Verification items for this drawing (mm, ordinates from the low corner). A direction names the side the tool comes from. Coordinates: 2 decimals unless noted, no trailing zeros. Order: outer loops, then holes, each group sorted by start corner. A loop starts at its lowest first (then second) coordinate and runs counter-clockwise, first axis right, second up. Notation, with made-up numbers: M -24.5,65.5 L -6.5,65.5 A23 cw -6.5,83.5 Z; hole C -22,26 d2. An arc over 180 degrees is marked long. Return JSON: item names as keys, results as strings. Group by question number.
1. Mould release check, pull along Z, two halves, no side actions. Record for the marked faces 3 and 4: +Z half, -Z half, draft (parallel to the pull), parting line (faces both ways), or undercut.
2. Section check B-B, the plane z = 13.9. Record the cut outline in (x, y).
3. Section check A-A, the plane x = 13.9. Record the cut outline in (y, z).
4. Material ranges on line 1 along Y through (x, z) = (10, 25.25); line 2 along X through (y, z) = (34, 14); line 3 along Y through (x, z) = (8.75, 20.75), recorded low to high.
5. Set-up check for the marked faces 1 and 2: record each of +Z, -Z, +X, -X, +Y, -Y from which the full face is reachable in a straight line by a thin tool's end or side.
6. Gauge pin test, flat ends, axial feed: pin 1 (4 mm diameter, centred on x = 8.24, z = 19.56, fed in from +Y); pin 2 (2.5 mm diameter, centred on x = 19.56, z = 8.24, fed in from -Y); pin 3 (4 mm diameter, centred on y = 6.5, z = 21.5, fed in from +X). Record the tip position at first contact, or that the pin passes through.
7. Section check C-C, the plane y = 14. Record the cut outline in (x, z), plus the area to 3 significant figures.
8. Section check D-D, the plane x = 24.75. Record the cut outline in (y, z).
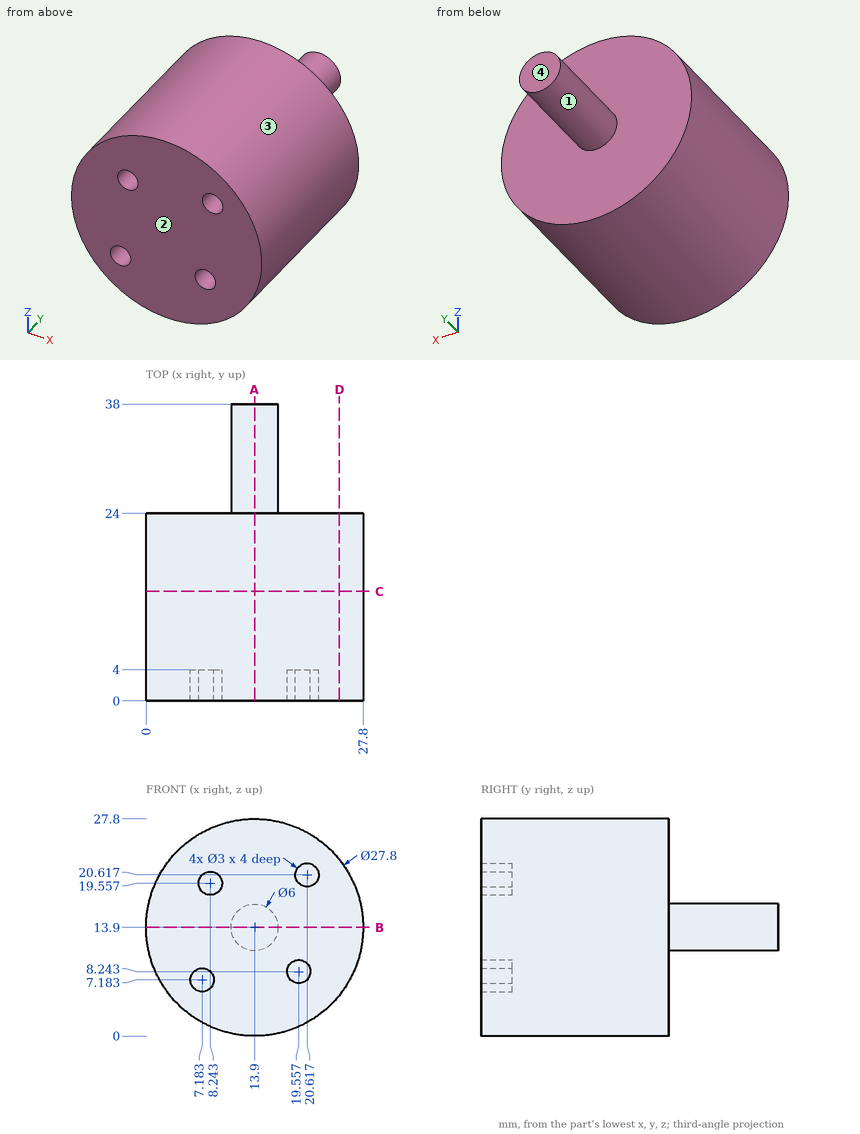
Answers follow:
{
 "1": {"face 3": "parting line", "face 4": "draft"},
 "2": {"outline": "M 0,0 L 27.8,0 L 27.8,24 L 16.9,24 L 16.9,38 L 10.9,38 L 10.9,24 L 0,24 Z"},
 "3": {"outline": "M 0,0 L 24,0 L 24,10.9 L 38,10.9 L 38,16.9 L 24,16.9 L 24,27.8 L 0,27.8 Z"},
 "4": {"line 1": "0 to 24", "line 2": "10.9 to 16.9", "line 3": "4 to 24"},
 "5": {"face 1": "+Y", "face 2": "+Z, -Z, +X, -X, -Y"},
 "6": {"pin 1": "y = 24", "pin 2": "y = 4", "pin 3": "x = 26.62"},
 "7": {"outline": "C 13.9,13.9 d27.8", "area": "607 mm^2"},
 "8": {"outline": "M 0,5.21 L 24,5.21 L 24,22.59 L 0,22.59 Z"}
}
